Can you work these out from the model? Positions are in its coordinate system, mm. Round coordinates to 2 decimals unless told otherwise and drop trailing zeros. Write each loop counter-clockwise with the first axis right and the second up, starting at its lowest first coordinate (ties: lowest second). Pieces come first, ordered by that corner, then holes.
Q1. I'm going to push flat-ended pins straight in: pin 1 Ø1 at (x, z) = (28.5, 1.5) entering from +Y; pin 2 Ø4 at (x, z) = (42, 2.5) entering from +Y. Where does each tip first touch, or does it pass through?
Q2. If we section it at A-A (x = 118): Please give me the cut outline in (y, z), plus the area to 3 significant figures.
Q3. Please list where these lines run through material, in increasing order: line 1 along Z through (x, y) = (153, -0.5); line 2 along Z through (x, y) = (35.5, 1).
Autodesk Inventor part; units mm, degrees
ref_plane "Płaszczyzna początkowa" through (0, 0, 0) normal (1, 0, 0) x (0, 1, 0)
ref_plane "XZ Plane" through (0, 0, 0) normal (0, 1, 0) x (-1, 0, 0)
ref_plane "XY Plane" through (0, 0, 0) normal (0, 0, 1) x (1, 0, 0)
sketch "Szkic główny" plane through (0, 0, 0) normal (0, 0, 1) x (1, 0, 0)
  line L0 (0, 0) -> (337, 0)
  line L1 (0, 0) -> (0, 4)
  line L2 (337, 4) -> (337, 0)
  line L3 (0, 4) -> (337, 4)
  dimension "d3" = 8
revolve "Obrót1" add sketch "Szkic główny" angle 360 about axis through (0, 0, 0) along (1, 0, 0)
thread "Gwint1"
chamfer "Faza1" distance 1 angle 45 2 edges at (0, -4, 0) (337, -4, 0)
sketch "Sketch3" plane through (337, 0, 0) normal (1, 0, 0) x (0, 0, -1)
  circle A0 centre (0, 0) radius 4
  circle A1 centre (0, 0) radius 3
  circle A2 centre (0, 0) radius 3
extrude "Extrusion1" add sketch "Sketch3" along normal blind 13 and the other way blind 1 contours A0 | A1
sketch "Boceto4" plane through (350, 0, 0) normal (1, 0, 0) x (0, 0, -1)
  circle A0 centre (0, 0) radius 3
  circle A1 centre (0, 0) radius 14.4832
extrude "Extrusión2" cut sketch "Boceto4" against normal blind 180 contours A0 | A1
properties part number "ACMEThread" material "Steel"
A:
1. pin 1: stops at y = 3.87
1. pin 2: stops at y = 3.97
2. outline: circle Ø8 at (0, 0)
2. area: 50.3 mm2
3. line 1: z = -3.97 to 3.97
3. line 2: z = -3.87 to 3.87
